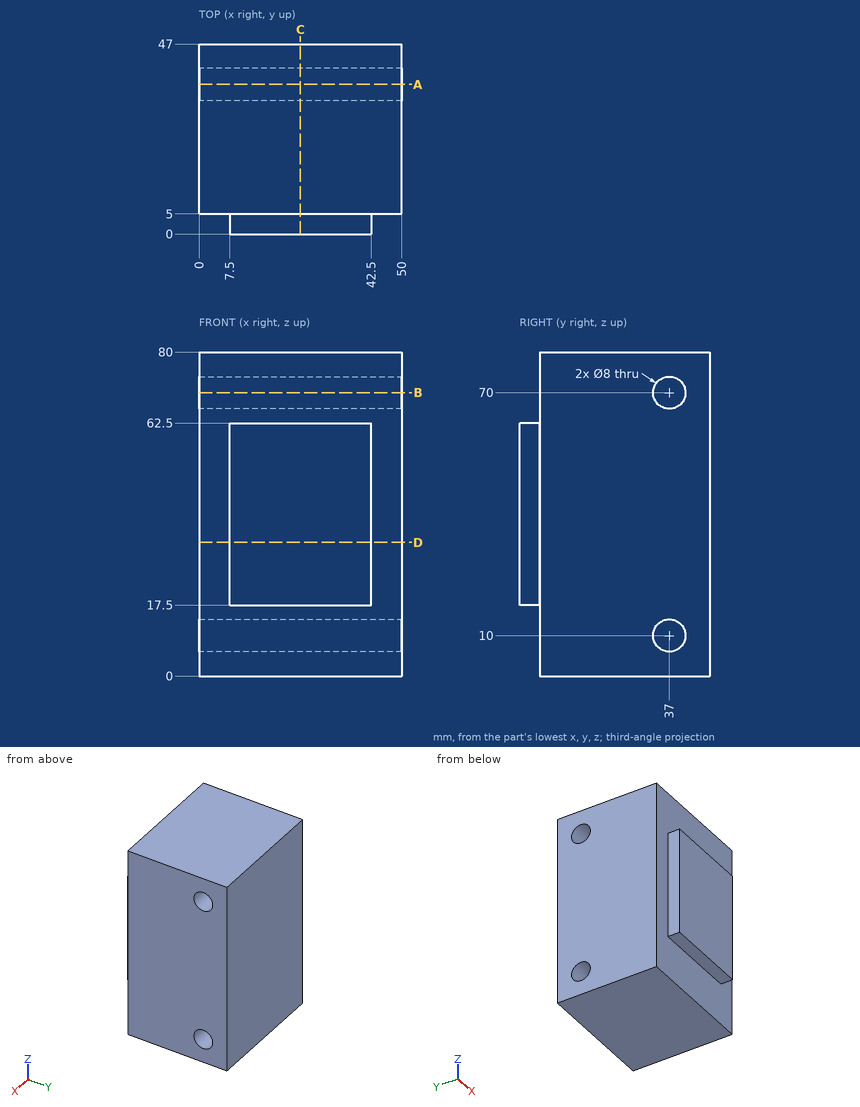
Here's the drawing with two shaded views (mm, measured from the low corner). I have some questions. Round coordinates to 2 decimals unless told otherwise and drop trailing zeros. Write each loop counter-clockwise with the first axis right and the second up, starting at its lowest first coordinate (ties: lowest second). Pieces come first, ordered by that corner, then holes. Notation, with made-up numbers: M 39,78.5 L 77,78.5 A22 cw 77,108.5 Z; hole C 39.25,38 d7. An arc over 180 degrees is marked long. Use CSV: the item, a comma, the result in double quotes.
(1) Imagine slicing it at B-B (z = 70). Write out the boundary of the cut face in (x, y), plus the area to 3 significant figures.
Check values:
outline,"M 0,5 L 50,5 L 50,33 L 0,33 Z; M 0,41 L 50,41 L 50,47 L 0,47 Z"
area,"1,700 mm^2"
(2) I need wall thicknesses on line 1 along Z through (x, y) = (5, 40); line 2 along Z through (x, y) = (17, 37.5); line 3 along Y through (x, z) = (18, 10). Which ranges of each line are inside material? Lowest first, please.
Check values:
line 1,"0 to 7.35, 12.65 to 67.35, 72.65 to 80"
line 2,"0 to 6.03, 13.97 to 66.03, 73.97 to 80"
line 3,"5 to 33, 41 to 47"
(3) I'm going to push flat-ended pins straight in: pin 1 (13 mm diameter, centred on y = 37, z = 70, fed in from -X); pin 2 (5.5 mm diameter, centred on y = 2, z = 29.5, fed in from -X); pin 3 (1.5 mm diameter, centred on y = 1.5, z = 37, fed in from +X); pin 4 (4 mm diameter, centred on x = 17.5, y = 2.5, fed in from -Z). Where does each tip first touch, or does it pass through?
Check values:
pin 1,"x = 0"
pin 2,"x = 7.5"
pin 3,"x = 42.5"
pin 4,"z = 17.5"
(4) Imagine slicing it at D-D (z = 33). Write out the boundary of the cut face in (x, y).
Check values:
outline,"M 0,5 L 7.5,5 L 7.5,0 L 42.5,0 L 42.5,5 L 50,5 L 50,47 L 0,47 Z"
(5) Imagine slicing it at A-A (y = 37). Write out the boundary of the cut face in (x, z).
Check values:
outline,"M 0,0 L 50,0 L 50,6 L 0,6 Z; M 0,14 L 50,14 L 50,66 L 0,66 Z; M 0,74 L 50,74 L 50,80 L 0,80 Z"
(6) Imagine slicing it at C-C (x = 25). Write out the boundary of the cut face in (y, z), plus the area to 3 significant figures.
Check values:
outline,"M 0,17.5 L 5,17.5 L 5,0 L 47,0 L 47,80 L 5,80 L 5,62.5 L 0,62.5 Z; hole C 37,10 d8; hole C 37,70 d8"
area,"3,480 mm^2"
